Check sheet for the drawn part. Datum: minimum x, y, z corner. Units: mm. A direction names the side the tool comes from. Give positions to 0.01 mm unless a question says otherwise; leave off trailing zeros. Order: outer loops, then holes, each group sorted by start corner. A loop starts at its lowest first (then second) coordinate and runs counter-clockwise, first axis right, second up.
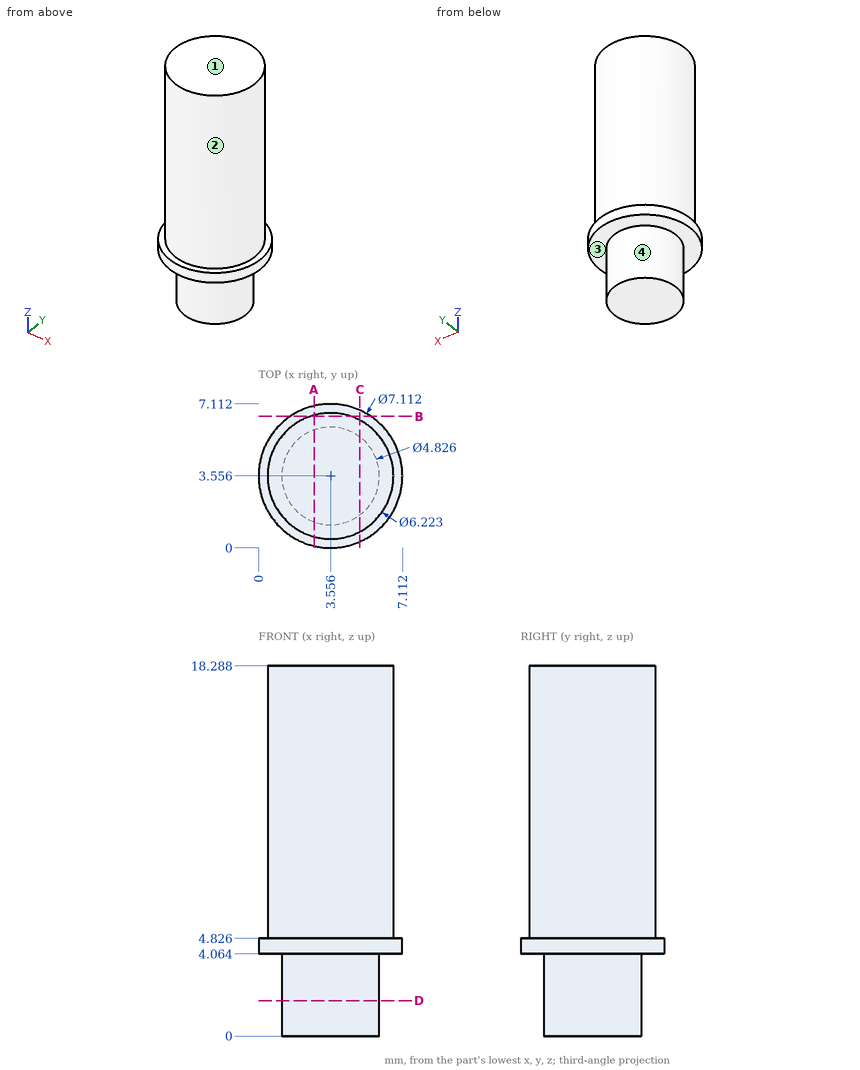
(1) Section check C-C, the plane x = 5. Enter the section's corners in (y, z), then the cut area to 3 significant figures.
Solved:
outline: (0.31, 4.06) - (1.62, 4.06) - (1.62, 0) - (5.49, 0) - (5.49, 4.06) - (6.81, 4.06) - (6.81, 4.83) - (6.31, 4.83) - (6.31, 18.29) - (0.8, 18.29) - (0.8, 4.83) - (0.31, 4.83) - close
area: 94.9 mm2
(2) Section check B-B, the plane y = 6.5. Enter the section's corners in (x, z), then the cut area to 3 significant figures.
Solved:
outline: (1.56, 4.06) - (5.55, 4.06) - (5.55, 4.83) - (4.56, 4.83) - (4.56, 18.29) - (2.55, 18.29) - (2.55, 4.83) - (1.56, 4.83) - close
area: 30.2 mm2
(3) Section check A-A, the plane x = 2.75. Enter the section's corners in (y, z).
Solved:
outline: (0.09, 4.06) - (1.28, 4.06) - (1.28, 0) - (5.83, 0) - (5.83, 4.06) - (7.02, 4.06) - (7.02, 4.83) - (6.56, 4.83) - (6.56, 18.29) - (0.55, 18.29) - (0.55, 4.83) - (0.09, 4.83) - close
(4) Release check for a two-part mould opening along X. For the marked faces 3 and 4 record: pulls with the +X half, pulls with the -X half, needs draft (parallel to the pull), parting line crosses it, or undercut.
Solved:
face 3: needs draft
face 4: parting line crosses it
(5) Scan lines: line 1 (Z direction, x = 6, y = 2); line 2 (X direction, y = 0.75, z = 13.25); line 3 (Y direction, x = 4, z = 15). Record each from-to range of solid material in increasing order.
Solved:
line 1: z = 4.06 to 18.29
line 2: x = 2.21 to 4.9
line 3: y = 0.48 to 6.64
(6) Go/stop test with flat-tipped pins: pin 1 (2 mm diameter, centred on x = 1.5, z = 12.5, fed in from +Y); pin 2 (3 mm diameter, centred on y = 6, z = 9, fed in from +X); pin 3 (4 mm diameter, centred on x = 4, z = 9, fed in from -Y). Record where each tip stops, or that it passes through.
Solved:
pin 1: stops at y = 6.48
pin 2: stops at x = 6.52
pin 3: stops at y = 0.44
(7) Section check D-D, the plane z = 1.75. Enter the section's corners in (x, y).
Solved:
outline: circle Ø4.83 at (3.56, 3.56)
(8) Set-up check for the marked faces 1 and 2: record each of +Z, -Z, +X, -X, +Y, -Y from which the full face is reachable in a straight line by a thin tool's end or side.
Solved:
face 1: +Z, +X, -X, +Y, -Y
face 2: +Z
